Job drawing, mm, ordinate dimensions from the low corner. One solid piece. Give positions to 0.01 mm unless a question says otherwise; leave off trailing zeros. Loops run counter-clockwise (first coordinate to the right, second up) from the corner with the lowest first, then second, coordinate; pieces in that order, holes last.
Item 1: Drop flat-ended pins along their axis: P1, Ø1.2, axis at x = 52.5, z = 3, coming from the -Y side; P2, Ø3, axis at x = 15.5, y = 64, coming from the -Z side; P3, Ø1, axis at y = 50, z = 0.5, coming from the +X side; P4, Ø1.2, axis at x = 24, z = 3, coming from the -Y side. Give the stop position or say it passes through.
Item 2: Saw through at A-A on y = 16. Give the cut face in (x, z), plus the area to 3 significant figures.
Item 3: Probe probe 1 along X at (y, z) = (97, 0.65); probe 2 along Y at (x, z) = (87, 3.5); probe 3 along Y at (x, z) = (31.5, 2). List the from-to ranges inside material, lowest first.
Item 4: Saw through at B-B on x = 15.5. Give the cut face in (y, z), plus the area to 3 significant figures.
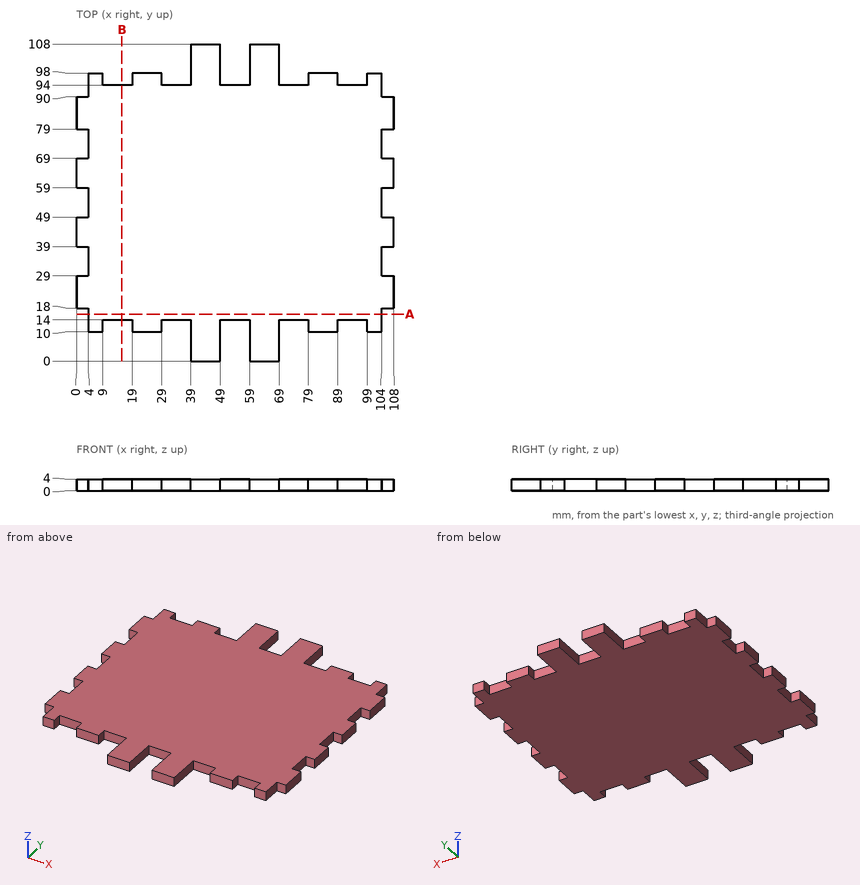
Results below:
1. P1: stops at y = 14
1. P2: stops at z = 0
1. P3: stops at x = 104
1. P4: stops at y = 10
2. outline: (4, 0) - (104, 0) - (104, 4) - (4, 4) - close
2. area: 400 mm2
3. probe 1: x = 4 to 9, 19 to 29, 39 to 49, 59 to 69, 79 to 89, 99 to 104
3. probe 2: y = 10 to 98
3. probe 3: y = 14 to 94
4. outline: (14, 0) - (94, 0) - (94, 4) - (14, 4) - close
4. area: 320 mm2
